Input: dimensioned drawing with shaded views. Units: mm. Origin: part minimum x, y, z. A direction names the side the tool comes from. Give positions to 0.01 mm unless a question says otherwise; leave off trailing zeros. Write each loop counter-clockwise with the first axis right and the second up, starting at its lowest first coordinate (ties: lowest second). Pieces come first, ordered by that corner, then holes. Notation, with made-up numbers: (56, 26) -> (96, 26) arc R12 cw to (96, 49) -> close; hole circle Ø9 at (34.5, -4). An arc over 180 degrees is marked (long way). Answer as a JSON object with one key per item and string values.
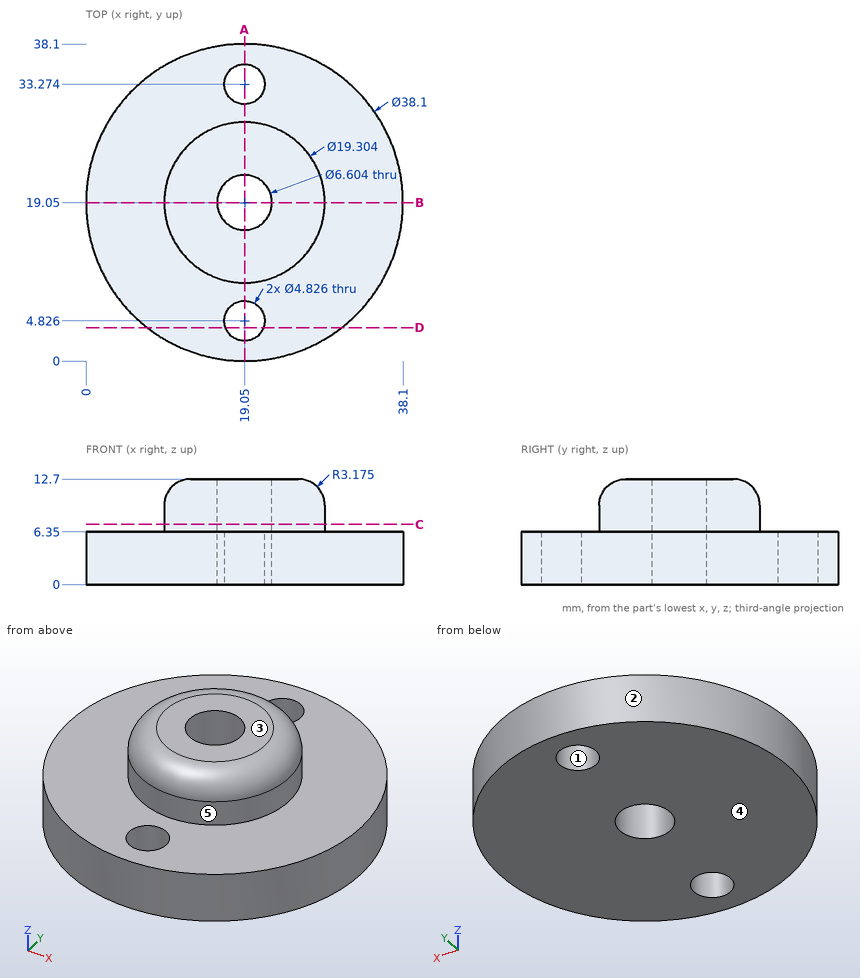
Q1. Cut plane C-C (z = 7.25). Return the cut outline in (x, y).
Values:
{"outline": "circle Ø19.3 at (19.05, 19.05); hole circle Ø6.6 at (19.05, 19.05)"}
Q2. First-contact query: P1, Ø11.5, axis at x = 19, y = 21.5, coming from the +Z side; P2, Ø1.5, axis at x = 13, y = 5.5, coming from the +Z side; P3, Ø6, axis at x = 19.05, y = 19.05, coming from the +Z side; P4, Ø5, axis at y = 15, z = 10.5, coming from the +X side. Flat tips, straight axial feed; report the tip coordinate or a pass-through.
Values:
{"P1": "z = 12.7", "P2": "z = 6.35", "P3": "through", "P4": "x = 28.55"}
Q3. Cut plane B-B (y = 19.05). Return the cut outline in (x, z) (3 decimals).
Values:
{"outline": "(0, 0) -> (15.748, 0) -> (15.748, 12.7) -> (12.573, 12.7) arc R3.175 ccw to (9.398, 9.525) -> (9.398, 6.35) -> (0, 6.35) -> close; (22.352, 0) -> (38.1, 0) -> (38.1, 6.35) -> (28.702, 6.35) -> (28.702, 9.525) arc R3.175 ccw to (25.527, 12.7) -> (22.352, 12.7) -> close"}
Q4. Material intervals for L1, parallel to Y at x = 19.05, z = 4.5; L2, parallel to Y at x = 19.05, z = 6.5, sorted ascending. Write a range as from..to.
Values:
{"L1": "0..2.41, 7.24..15.75, 22.35..30.86, 35.69..38.1", "L2": "9.4..15.75, 22.35..28.7"}
Q5. Set-up query: the marked faces 4 and 5. Return all of +Z, -Z, +X, -X, +Y, -Y with unobstructed straight access to the full face (end or side cutting, diameter ignored); none if empty.
Values:
{"face 4": "-Z, +X, -X, +Y, -Y", "face 5": "+Z"}
Q6. Mould query, pull axis X, two halves, no side actions, for the marked faces 1, 2 and 3. Classes: pulls with the +X half, pulls with the -X half, needs draft (parallel to the pull), parting line crosses it, or undercut.
Values:
{"face 1": "undercut", "face 2": "parting line crosses it", "face 3": "needs draft"}
Q7. Cut plane A-A (x = 19.05). Return the cut outline in (y, z) (3 decimals), and give its area (3 significant figures).
Values:
{"outline": "(0, 0) -> (2.413, 0) -> (2.413, 6.35) -> (0, 6.35) -> close; (7.239, 0) -> (15.748, 0) -> (15.748, 12.7) -> (12.573, 12.7) arc R3.175 ccw to (9.398, 9.525) -> (9.398, 6.35) -> (7.239, 6.35) -> close; (22.352, 0) -> (30.861, 0) -> (30.861, 6.35) -> (28.702, 6.35) -> (28.702, 9.525) arc R3.175 ccw to (25.527, 12.7) -> (22.352, 12.7) -> close; (35.687, 0) -> (38.1, 0) -> (38.1, 6.35) -> (35.687, 6.35) -> close", "area": "215 mm²"}
Q8. Cut plane D-D (y = 4). Return the cut outline in (x, z), and give its area (3 significant figures).
Values:
{"outline": "(7.37, 0) -> (16.78, 0) -> (16.78, 6.35) -> (7.37, 6.35) -> close; (21.32, 0) -> (30.73, 0) -> (30.73, 6.35) -> (21.32, 6.35) -> close", "area": "120 mm²"}
